Part model, mm, in its own coordinate system. Face numbers are marked on the shaded views. Round coordinates to 2 decimals unless told otherwise and drop trailing zeros. Write each loop counter-clockwise with the first axis right and the second up, starting at its lowest first coordinate (ties: lowest second). Pieces come first, ordered by that corner, then holes. Notation, with made-up numbers: M -31,-1.75 L -2,-1.75 A20 ccw -2,13.25 Z; hole C -35.75,43 d3. An arc over 180 degrees is marked long. Answer as a JSON object with one key per item and string values. Group by question number.
1. Band-saw the part on D-D, the plane x = -12.5. Write the cut outline in (y, z).
2. Two-plate mould, pull along Z, no slides. Class the marked faces 1, 2, 3 and 4: +Z half, -Z half, draft (parallel to the pull), parting line (faces both ways), or undercut.
3. Band-saw the part on B-B, the plane z = -2.5. Write the cut outline in (x, y), plus the area to 3 significant figures.
4. Band-saw the part on C-C, the plane y = -0.35. Write the cut outline in (x, z), plus the area to 3 significant figures.
5. Band-saw the part on A-A, the plane y = -2.3. Write the cut outline in (x, z).
6. Drill centre lines: line 1 (Z direction, x = -12.5, y = -1.4); line 2 (X direction, y = -2.25, z = 5); line 3 (Y direction, x = 1, z = -0.25). Where is each one in solid material? Low to high. Write a range as from..to.
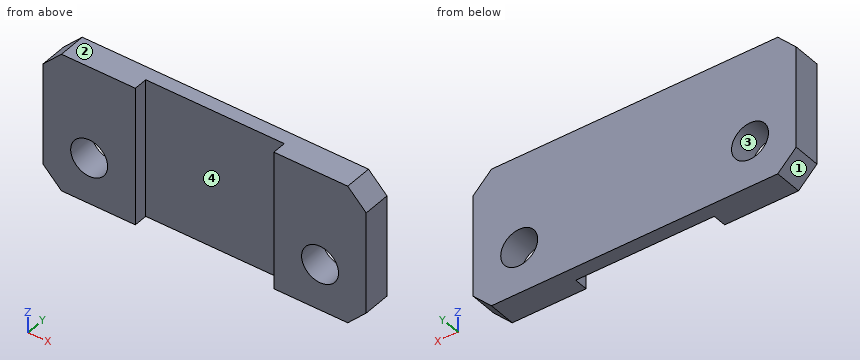
from build123d import *

# Parameters (mm, degrees)
F0_W     = 35
F0_H     = 15
F1_DEPTH = 4.5
F2_W     = 15
F2_H     = 1.5
F3_DEPTH = 15.001
F4_R     = 2
F5_DEPTH = 10
F6_SIZE  = 2
F7_W     = 39.253565
F7_H     = 1.5
F8_DEPTH = 15.001


with BuildPart() as f1:
    # F0 (on Front) → F1 (new body)
    with BuildSketch(Plane.XZ):
        Rectangle(F0_W, F0_H)
    extrude(amount=F1_DEPTH)

    # F2 (on face) → F3 (cut, through all)
    with BuildSketch(Plane.XY.offset(7.5)):
        with Locations((0, -2.25)):
            Rectangle(F2_W, F2_H)
    extrude(amount=-F3_DEPTH, mode=Mode.SUBTRACT)

    # F4 (on face) → F5 (cut)
    with BuildSketch(Plane.XZ.offset(4.5)):
        with Locations((12.5, -2.5)):
            Circle(F4_R)
        with Locations((-12.5, -2.5)):
            Circle(F4_R)
    extrude(amount=-F5_DEPTH, mode=Mode.SUBTRACT)

    # F6
    f6_edges = [f1.edges().sort_by_distance(p)[0] for p in [
        (-17.5, -2.25, 7.5),
        (17.5, -2.25, 7.5),
        (17.5, -2.25, -7.5),
        (-17.5, -2.25, -7.5),
    ]]
    chamfer(f6_edges, length=F6_SIZE)

    # F7 (on face) → F8 (cut, through all)
    with BuildSketch(Plane.XY.offset(7.5)):
        with Locations((0.571815, -3.75)):
            Rectangle(F7_W, F7_H)
    extrude(amount=-F8_DEPTH, mode=Mode.SUBTRACT)


solid = f1.part
Worked answers:
{
 "1": {"outline": "M -3,-7.5 L 0,-7.5 L 0,-4.5 L -3,-4.5 Z; M -3,-0.5 L 0,-0.5 L 0,7.5 L -3,7.5 Z"},
 "2": {"face 1": "-Z half", "face 2": "+Z half", "face 3": "undercut", "face 4": "draft"},
 "3": {"outline": "M -17.5,-3 L -14.5,-3 L -14.5,0 L -17.5,0 Z; M -10.5,-3 L -7.5,-3 L -7.5,-1.5 L 7.5,-1.5 L 7.5,-3 L 10.5,-3 L 10.5,0 L -10.5,0 Z; M 14.5,-3 L 17.5,-3 L 17.5,0 L 14.5,0 Z", "area": "58.5 mm^2"},
 "4": {"outline": "M -17.5,-5.5 L -15.5,-7.5 L 15.5,-7.5 L 17.5,-5.5 L 17.5,5.5 L 15.5,7.5 L -15.5,7.5 L -17.5,5.5 Z; hole C -12.5,-2.5 d4; hole C 12.5,-2.5 d4", "area": "492 mm^2"},
 "5": {"outline": "M -17.5,-5.5 L -15.5,-7.5 L -7.5,-7.5 L -7.5,7.5 L -15.5,7.5 L -17.5,5.5 Z; M 7.5,-7.5 L 15.5,-7.5 L 17.5,-5.5 L 17.5,5.5 L 15.5,7.5 L 7.5,7.5 Z; hole C -12.5,-2.5 d4; hole C 12.5,-2.5 d4"},
 "6": {"line 1": "z = -7.5..-4.5, -0.5..7.5", "line 2": "x = -17.5..-7.5, 7.5..17.5", "line 3": "y = -1.5..0"}
}
